Autodesk Inventor part; units mm, degrees
ref_plane "YZ Plane" through (0, 0, 0) normal (1, 0, 0) x (0, 1, 0)
ref_plane "XZ Plane" through (0, 0, 0) normal (0, 1, 0) x (-1, 0, 0)
ref_plane "XY Plane" through (0, 0, 0) normal (0, 0, 1) x (1, 0, 0)
sketch "Sketch1" plane through (0, 0, 0) normal (0, 0, 1) x (1, 0, 0)
  line L0 (0, 0) -> (18, 0) construction
  line L1 (18, -55) -> (0, -55) construction
  line L2 (-0.2, 0) -> (4, 0)
  line L3 (18.2, 0) -> (18.2, -55)
  line L4 (18.2, -55) -> (14, -55)
  line L5 (-0.2, -55) -> (-0.2, 0)
  line L6 (14, 0) -> (14, -5)
  line L7 (14, -5) -> (4, -5)
  line L8 (4, -5) -> (4, 0)
  line L9 (14, 0) -> (18.2, 0)
  line L10 (14, -55) -> (14, -49.9766)
  line L11 (14, -49.9766) -> (4, -49.9766)
  line L12 (4, -49.9766) -> (4, -55)
  line L13 (4, -55) -> (-0.2, -55)
  point P0 (1, -55)
  point P1 (16.8146, 0)
  point P2 (4, -2.5)
  point P3 (4, -52.4883)
  point P4 (14, -52.4883)
  point P5 (14, -2.5)
  dimension "d33" = 18.4
  dimension "d34" = 0.2
  dimension "d35" = 4.2
  dimension "d36" = 4.2
  dimension "d37" = 5
  dimension "d38" = 0
  dimension "d39" = 5.0234
  dimension "d40" = 0
extrude "Extrusion1" add sketch "Sketch1" along normal blind 5
sketch "Sketch3" plane through (0, 0, 5) normal (0, 0, 1) x (1, 0, 0)
  line L0 (-0.2, 0) -> (-0.2, -55)
  circle A0 centre (9, -15) radius 1.5
  line L1 (4, 0) -> (-0.2, 0)
  point P0 (0, 0)
  point P1 (1, -55)
  dimension "d21" = 3
  dimension "d25" = 9.2
  dimension "d41" = 15
hole "Hole2" at (9, -15, 5) direction (0, 0, -1) diameter 3 depth 8 tip angle 118
equation "\"d26\" = d21"
properties part number "Z-Kettenhalter"
Model file for the job. Use its own axes, mm. A direction names the side the tool comes from. Coordinates: 2 decimals unless noted, no trailing zeros. Write each loop counter-clockwise with the first axis right and the second up, starting at its lowest first coordinate (ties: lowest second). Pieces come first, ordered by that corner, then holes. Notation, with made-up numbers: (-14.75, 89.25) -> (-0.75, 89.25) arc R30 ccw to (-0.75, 127.25) -> close; hole circle Ø5 at (9.25, -24). An arc over 180 degrees is marked (long way). One line per item, written item: value. Start each with the question number.
1) Which spindle directions (+Z, -Z, +X, -X, +Y, -Y) get a long thin tool onto all of the face, cutting with end or side? Do faces 1 (the face through (4, -52, 2)), 2 (the face through (2, -55, 2)), 3 (the face through (9, -5, 2)). Say none if no direction does.
2) Flat gauge pins, fed straight in: pin 1 Ø4 at (x, y) = (9, -15) entering from -Z; pin 2 Ø2.5 at (x, z) = (8.5, 1.5) entering from -Y. Where does each tip first touch, or does it go through?
3) Slice it at D-D on x = 4.75. Write the cut outline in (y, z).
4) Pull direction X, two halves, no side cores. Call faces 4 (the face through (18.2, -27, 2)), 5 (the face through (16, 0, 2)), 6 (the face through (14, -53, 2)): +X half, -X half, draft (parallel to the pull), parting line (faces both ways), or undercut.
5) Probe probe 1 along Y at (x, z) = (9, 3.7); probe 2 along X at (y, z) = (-15, 3.25); probe 3 along Y at (x, z) = (6, 2.05). List the from-to ranges inside material, lowest first.
6) Slice it at C-C on z = 1.2. Write the cut outline in (x, y), then the cut area to 3 significant figures.
7) Slice it at A-A on x = 9. Write the cut outline in (y, z), then the cut area to 3 significant figures.
8) Slice it at B-B on y = -15. Write the cut outline in (x, z).
Answers follow:
1. face 1: +Z, -Z, -Y
1. face 2: +Z, -Z, +X, -X, -Y
1. face 3: +Z, -Z, +Y
2. pin 1: z = 0
2. pin 2: y = -49.98
3. outline: (-49.98, 0) -> (-5, 0) -> (-5, 5) -> (-49.98, 5) -> close
4. face 4: +X half
4. face 5: draft
4. face 6: undercut
5. probe 1: -49.98 to -16.5, -13.5 to -5
5. probe 2: -0.2 to 7.5, 10.5 to 18.2
5. probe 3: -49.98 to -5
6. outline: (-0.2, -55) -> (4, -55) -> (4, -49.98) -> (14, -49.98) -> (14, -55) -> (18.2, -55) -> (18.2, 0) -> (14, 0) -> (14, -5) -> (4, -5) -> (4, 0) -> (-0.2, 0) -> close; hole circle Ø3 at (9, -15)
6. area: 905 mm2
7. outline: (-49.98, 0) -> (-16.5, 0) -> (-16.5, 5) -> (-49.98, 5) -> close; (-13.5, 0) -> (-5, 0) -> (-5, 5) -> (-13.5, 5) -> close
7. area: 210 mm2
8. outline: (-0.2, 0) -> (7.5, 0) -> (7.5, 5) -> (-0.2, 5) -> close; (10.5, 0) -> (18.2, 0) -> (18.2, 5) -> (10.5, 5) -> close
